Study the drawing (mm; zero at the part's minimum x, y, z) and answer. Coordinates: 2 decimals unless noted, no trailing zeros. Order: outer loops, then holes, each group sorted by start corner. A loop starts at its lowest first (then second) coordinate and runs counter-clockwise, first axis right, second up. Notation, with made-up numbers: M 15,76 L 71,76 A33 ccw 71,109 Z; hole C 26.25,-17.75 d6. An arc over 180 degrees is marked long. One line per item, written item: value. Start each with the question number.
Q1. Determine the mould class of the marked faces 1, 2 and 3 for opening direction X: pulls with the +X half, pulls with the -X half, needs draft (parallel to the pull), parting line crosses it, or undercut.
Q2. The part is cut by section A-A on y = 4.25. Give the vertices of the cut face in (x, z).
Q3. The part is cut by section B-B on z = 14.98. Give the vertices of the cut face in (x, y).
Q4. The part is cut by section C-C on x = 12. Give the vertices of the cut face in (y, z).
Q5. Straight lines are drawn through the part: line 1 along X through (y, z) = (1.05, 14.98); line 2 along Z through (x, y) = (16.25, 4.05); line 3 along Z through (x, y) = (14, 1.35). For each, find the intervals that lie inside material, in ascending order. Write a range as [from, to].
Q6. The part is cut by section D-D on z = 26.5. Give the vertices of the cut face in (x, y), then the cut area to 3 significant figures.
Q7. Each of these flat-tipped pins is pushed along its axis until it touches: pin 1 Ø2.5 at (x, z) = (14.98, 25.98) entering from -Y; pin 2 Ø2 at (y, z) = (2, 19.5) entering from +X; pin 3 Ø1.5 at (x, y) = (16.5, 3.5) entering from +Z; pin 4 Ø1.5 at (x, y) = (5.5, 2) entering from -Z. Where does it stop, or does it pass through?
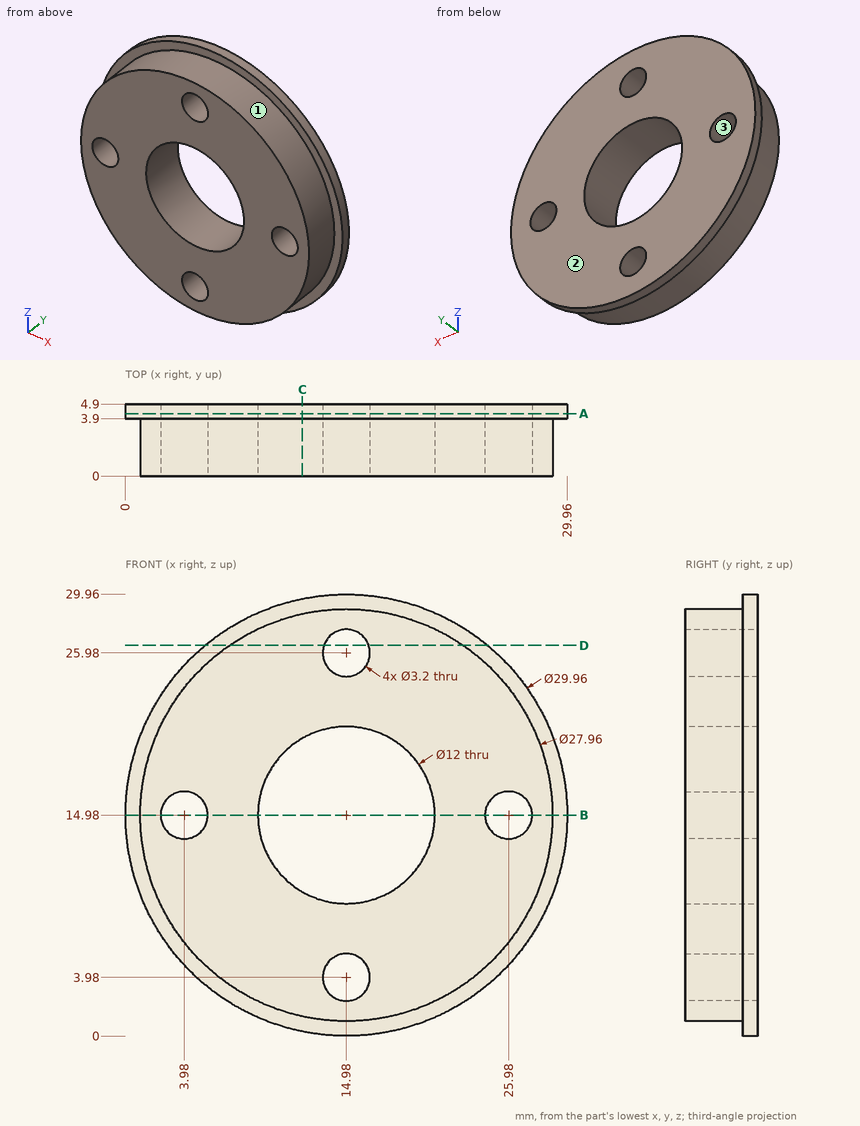
Output:
1. face 1: parting line crosses it
1. face 2: needs draft
1. face 3: undercut
2. outline: C 14.98,14.98 d29.96; hole C 3.98,14.98 d3.2; hole C 14.98,14.98 d12; hole C 14.98,3.98 d3.2; hole C 14.98,25.98 d3.2; hole C 25.98,14.98 d3.2
3. outline: M 0,3.9 L 1,3.9 L 1,0 L 2.38,0 L 2.38,4.9 L 0,4.9 Z; M 5.58,0 L 8.98,0 L 8.98,4.9 L 5.58,4.9 Z; M 20.98,0 L 24.38,0 L 24.38,4.9 L 20.98,4.9 Z; M 27.58,0 L 28.96,0 L 28.96,3.9 L 29.96,3.9 L 29.96,4.9 L 27.58,4.9 Z
4. outline: M 0,1.32 L 3.9,1.32 L 3.9,0.3 L 4.9,0.3 L 4.9,9.77 L 0,9.77 Z; M 0,20.19 L 4.9,20.19 L 4.9,29.66 L 3.9,29.66 L 3.9,28.64 L 0,28.64 Z
5. line 1: x = [1, 2.38], [5.58, 8.98], [20.98, 24.38], [27.58, 28.96]
5. line 2: z = [0.05, 3.01], [4.95, 9.12], [20.84, 25.01], [26.95, 29.91]
5. line 3: z = [1.03, 2.72], [5.24, 9.06], [20.9, 24.72], [27.24, 28.93]
6. outline: M 5.4,3.9 L 7.06,3.9 L 7.06,0 L 13.47,0 L 13.47,4.9 L 5.4,4.9 Z; M 16.49,0 L 22.9,0 L 22.9,3.9 L 24.56,3.9 L 24.56,4.9 L 16.49,4.9 Z
6. area: 66.1 mm^2
7. pin 1: passes through
7. pin 2: stops at x = 28.51
7. pin 3: stops at z = 29.93
7. pin 4: stops at z = 4.06
